The listing builds one solid part. Answer for the finished solid, in the listing's coordinates (mm). A direction names the side the tool comes from. Round coordinates to 2 decimals unless told otherwise and drop trailing zeros. Write each loop counter-clockwise with the first axis right and the second up, starting at its lowest first coordinate (ties: lowest second). Pieces come first, ordered by that corner, then holes.
(1) Find the intervals of material crossed by probe 1 along Z at (x, y) = (7.75, 10.5); probe 2 along Y at (x, z) = (-1.25, 86.5), in increasing order.
(2) For faces 1 (the face through (4, 0, 155)), 2 (the face through (-5, 1, 10)), 3 (the face through (-5, -4, 160)), determine the directions among +Z, -Z, +X, -X, +Y, -Y from which every point of the face is accessible in a straight line to the end or side of a thin tool.
(3) Each of these flat-tipped pins is pushed along its axis until it touches: pin 1 Ø1.5 at (x, z) = (3.5, 130.5) entering from +Y; pin 2 Ø1.5 at (y, z) = (-37.5, 106) entering from +X; pin 3 Ø4 at (x, y) = (5, -26.5) entering from -Z. Where does it stop, or does it pass through?
(4) A cutting plane is placed at C-C, the plane y = -36.5. Give the vertices of the cut face in (x, z), and give its area (3 significant figures).
(5) The mould has two halves that part along X. Classify faces 4 (the face through (0, -30, 155)), 5 (the face through (0, 30, 5)), 6 (the face through (-10, -42, 80)), 7 (the face through (0, 40, 5)): +X half, -X half, draft (parallel to the pull), parting line (faces both ways), or undercut.
(6) A cutting plane is placed at A-A, the plane y = -25.5. Give the vertices of the cut face in (x, z).
(7) A cutting plane is placed at D-D, the plane x = -7.75. Give the vertices of the cut face in (y, z).
(8) A cutting plane is placed at B-B, the plane x = 1.25. Give the vertices of the cut face in (y, z), and give its area (3 significant figures).
from build123d import *

# Parameters (mm, degrees)
ESBO_O1_W                = 20
ESBO_O1_H                = 80
ESBO_O1_W_2              = 8
ESBO_O1_H_2              = 60
RESSALTO_EXTRUS_O1_DEPTH = 10
ESBO_O1_4_W              = 20
ESBO_O1_4_H              = 10
RESSALTO_EXTRUS_O3_DEPTH = 80


with BuildPart() as part:
    # Esboço1 → Ressalto-extrusão1 (new body)
    with BuildSketch(Plane.XY):
        Rectangle(ESBO_O1_W, ESBO_O1_H)
        Rectangle(ESBO_O1_W_2, ESBO_O1_H_2, mode=Mode.SUBTRACT)
    ressalto_extrus_o1 = extrude(amount=RESSALTO_EXTRUS_O1_DEPTH)

    # Esboço1<4> → Ressalto-extrusão3 (add)
    with BuildSketch(Plane.XY):
        with Locations((0, -45)):
            Rectangle(ESBO_O1_4_W, ESBO_O1_4_H)
    ressalto_extrus_o3 = extrude(amount=RESSALTO_EXTRUS_O3_DEPTH)

    # Espelhar2: Ressalto-extrusão1, Ressalto-extrusão3 across plane
    add(ressalto_extrus_o1.mirror(Plane.XY.offset(80)))
    add(ressalto_extrus_o3.mirror(Plane.XY.offset(80)))


solid = part.part
Solutions:
1. probe 1: z = 0 to 10, 150 to 160
1. probe 2: y = -50 to -40
2. face 1: +Z, -Z
2. face 2: +X, -X, +Y
2. face 3: +Z, +X, -X, +Y, -Y
3. pin 1: stops at y = -40
3. pin 2: passes through
3. pin 3: stops at z = 0
4. outline: (-10, 0) - (10, 0) - (10, 10) - (-10, 10) - close; (-10, 150) - (10, 150) - (10, 160) - (-10, 160) - close
4. area: 400 mm2
5. face 4: undercut
5. face 5: undercut
5. face 6: -X half
5. face 7: draft
6. outline: (-10, 0) - (-4, 0) - (-4, 10) - (-10, 10) - close; (-10, 150) - (-4, 150) - (-4, 160) - (-10, 160) - close; (4, 0) - (10, 0) - (10, 10) - (4, 10) - close; (4, 150) - (10, 150) - (10, 160) - (4, 160) - close
7. outline: (-50, 0) - (40, 0) - (40, 10) - (-40, 10) - (-40, 150) - (40, 150) - (40, 160) - (-50, 160) - close
8. outline: (-50, 0) - (-30, 0) - (-30, 10) - (-40, 10) - (-40, 150) - (-30, 150) - (-30, 160) - (-50, 160) - close; (30, 0) - (40, 0) - (40, 10) - (30, 10) - close; (30, 150) - (40, 150) - (40, 160) - (30, 160) - close
8. area: 2,000 mm2
